Could you check a few things on this drawing? It's one solid part, dimensions in mm from its lowest x, y, z. A direction names the side the tool comes from. Give positions to 0.01 mm unless a question says otherwise; leave off trailing zeros. Loops run counter-clockwise (first coordinate to the right, second up) from the corner with the lowest first, then second, coordinate; pieces in that order, holes last.
1. Imagine slicing it at A-A (x = 19.05). List the corners of the cut face in (y, z) for me (3 decimals), plus the area to 3 significant figures.
2. Imagine slicing it at B-B (y = 38.1). Count the separate pieces of the cut face and the enclosed holes in it, plus the area to 3 significant figures.
3. For P1, Ø6, axis at x = 4, y = 9.5, coming from the -Z side; P2, Ø10, axis at y = 14.5, z = 28, coming from the +X side; P3, Ø2, axis at y = 12.5, z = 17, coming from the +X side; P4, Ø14.5, axis at y = 15, z = 21, coming from the +X side (3 decimals), each with a flat end and sliding along its axis, tell me the tip position at first contact or that it passes through.
4. For the marked faces 1 and 2, which set-ups out of +Z, -Z, +X, -X, +Y, -Y let a thin tool reach every point of the face, with its end or its side?
5. I need wall thicknesses on line 1 along Y through (x, z) = (1.25, 19.05) (3 decimals); line 2 along X through (y, z) = (21, 20) (3 decimals); line 3 along Z through (x, y) = (7.5, 14.5) (3 decimals). Which ranges of each line are inside material? Lowest first, please.
6. Imagine slicing it at C-C (z = 17.5). List the corners of the cut face in (x, y) for me (3 decimals).
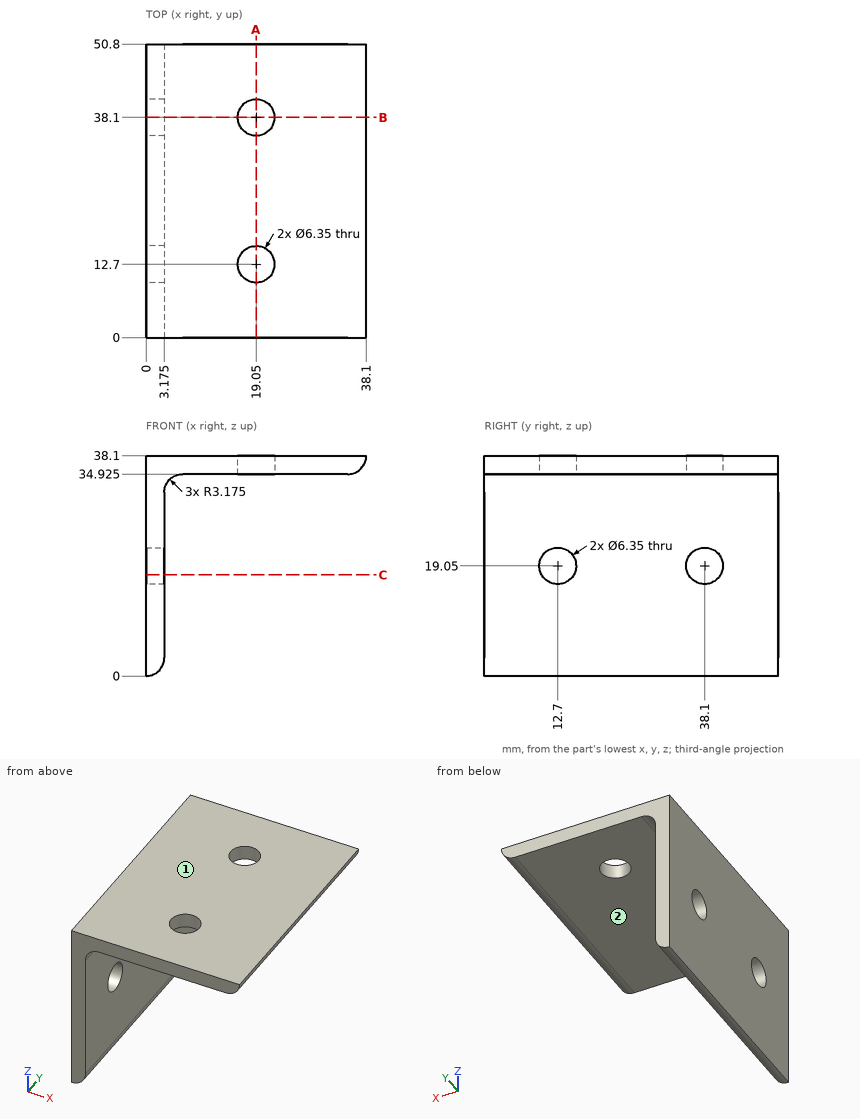
Derived:
1. outline: (0, 34.925) - (9.525, 34.925) - (9.525, 38.1) - (0, 38.1) - close; (15.875, 34.925) - (34.925, 34.925) - (34.925, 38.1) - (15.875, 38.1) - close; (41.275, 34.925) - (50.8, 34.925) - (50.8, 38.1) - (41.275, 38.1) - close
1. area: 121 mm2
2. separate pieces: 3
2. enclosed holes: 0
2. area: 189 mm2
3. P1: stops at z = 0.16
3. P2: stops at x = 3.43
3. P3: passes through
3. P4: stops at x = 3.175
4. face 1: +Z, +X, -X, +Y, -Y
4. face 2: -Z, +X, +Y, -Y
5. line 1: y = 0 to 9.525, 15.875 to 34.925, 41.275 to 50.8
5. line 2: x = 0 to 3.175
5. line 3: z = 34.925 to 38.1
6. outline: (0, 0) - (3.175, 0) - (3.175, 9.929) - (0, 9.929) - close; (0, 15.471) - (3.175, 15.471) - (3.175, 35.329) - (0, 35.329) - close; (0, 40.871) - (3.175, 40.871) - (3.175, 50.8) - (0, 50.8) - close
